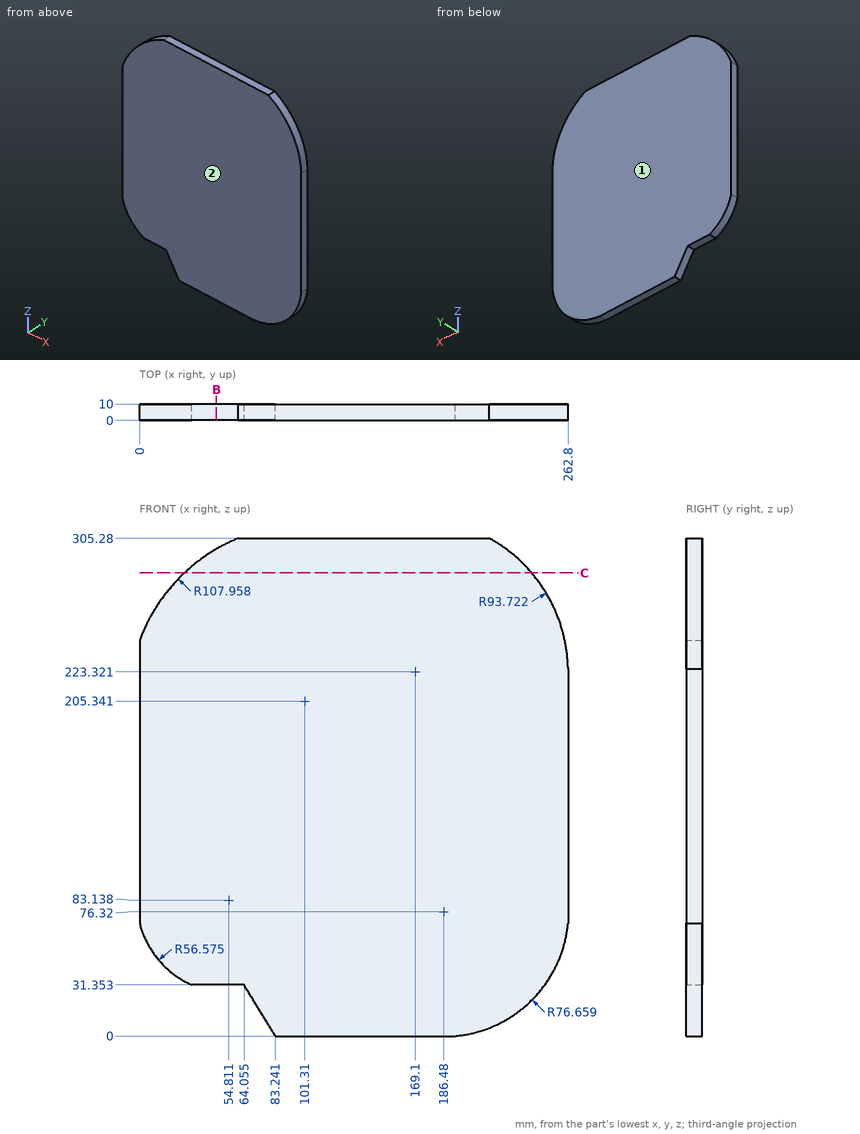
Source: three-view drawing plus pictorial views. Frame: mm from the lowest corner of the part. Coordinates: 2 decimals unless noted, no trailing zeros. Write each loop counter-clockwise with the first axis right and the second up, starting at its lowest first coordinate (ties: lowest second). Pieces come first, ordered by that corner, then holes. Notation, with made-up numbers: (-29, 87.5) - (-4, 87.5) arc R22 cw to (-4, 111.5) - close; hole circle Ø6 at (15, -28.5). An arc over 180 degrees is marked (long way). Return JSON: item names as keys, results as strings.
Item 1: Section query C-C (z = 284). Output: boundary loops of the cut face in (x, y).
Completed:
{"outline": "(27.37, 0) - (240.53, 0) - (240.53, 10) - (27.37, 10) - close"}
Item 2: Pin query (flat end, axial travel): pin 1 Ø2 at (x, y) = (226, 6.5) entering from +Z; pin 2 Ø3 at (x, y) = (41, 7) entering from -Z; pin 3 Ø3 at (y, z) = (2.5, 232.5) entering from +X. Return the tip coordinate at first contact, or that it passes through.
Completed:
{"pin 1": "stops at z = 298.55", "pin 2": "stops at z = 31.35", "pin 3": "stops at x = 262.51"}
Item 3: Section query B-B (x = 47). Output: boundary loops of the cut face in (y, z).
Completed:
{"outline": "(0, 31.35) - (10, 31.35) - (10, 298.64) - (0, 298.64) - close"}
Item 4: Pull-direction query (Y, two-part tool) for the marked faces 1 and 2; classes: +Y half, -Y half, draft (parallel to the pull), parting line (faces both ways), or undercut.
Completed:
{"face 1": "+Y half", "face 2": "-Y half"}
Item 5: Line query: L1, parallel to X at y = 3.75, z = 68 (1 decimal); L2, parallel to X at y = 8.25, z = 234; L3, parallel to Z at x = 226, y = 7.25 (1 decimal). Output: solid intervals per line, ascending.
Completed:
{"L1": "x = 0.3 to 262.7", "L2": "x = 0 to 262.21", "L3": "z = 10.6 to 297.8"}
